Read the model definition and answer for the solid it produces. Units are mm, in the model's axes. A direction names the side the tool comes from. Coordinates: 2 decimals unless noted, no trailing zeros. Loops run counter-clockwise (first coordinate to the right, second up) from the corner with the lowest first, then second, coordinate; pieces in that order, holes last. Notation, with made-up numbers: (-25, -24) - (-2, -24) arc R4 ccw to (-2, -20) - close; hole circle Ø4 at (-2.75, -7). An arc over 180 degrees is marked (long way). One line per item, written item: value. Start each with the question number.
from build123d import *

# Parameters (mm, degrees)
SKETCH_1_W          = 41.5
SKETCH_1_H          = 16
EXTRUDE_1_DEPTH     = 28.5
FILLET_1_R          = 1
FILLET_2_R          = 0.5
CUT_EXTRUDE_START   = -0.5
CUT_EXTRUDE_1_DEPTH = 0.5
SKETCH_4_R          = 0.5
EXTRUDE_2_DEPTH     = 6


with BuildPart() as part:
    # Эскиз1 → Бобышка-Вытянуть1 (new body)
    with BuildSketch(Plane(origin=(0, 0, 0), x_dir=(1, 0, 0), z_dir=(0, 1, 0))):
        Rectangle(SKETCH_1_W, SKETCH_1_H)
    extrude(amount=EXTRUDE_1_DEPTH)

    # Скругление1
    fillet_1_edges = [part.edges().sort_by_distance(p)[0] for p in [
        (20.75, 14.25, 8),
        (-20.75, 14.25, 8),
        (-20.75, 14.25, -8),
        (20.75, 14.25, -8),
    ]]
    fillet(fillet_1_edges, radius=FILLET_1_R)

    # Скругление2
    fillet_2_edges = [part.edges().sort_by_distance(p)[0] for p in [
        (0, 28.5, -8),
        (20.75, 28.5, 0),
        (-20.75, 28.5, 0),
        (0, 28.5, 8),
        (-20.457106781, 28.5, 7.707106781),
        (-20.457106781, 28.5, -7.707106781),
        (20.457106781, 28.5, 7.707106781),
        (20.457106781, 28.5, -7.707106781),
    ]]
    fillet(fillet_2_edges, radius=FILLET_2_R)

    # Эскиз3 → Вырез-Вытянуть1 (cut)
    with BuildSketch(Plane.XZ.offset(CUT_EXTRUDE_START)):
        with BuildLine():
            Line((-10.920111581, 7.5), (-10.920111581, 8))
            Line((-10.920111581, 8), (-19.75, 8))
            ThreePointArc((-19.75, 8), (-20.457106781, 7.707106781), (-20.75, 7))
            Line((-20.75, 7), (-20.75, -7))
            ThreePointArc((-20.75, -7), (-20.457106781, -7.707106781), (-19.75, -8))
            Line((-19.75, -8), (-10.920111581, -8))
            Line((-10.920111581, -8), (-10.920111581, -7.5))
            Line((-10.920111581, -7.5), (-8.050796548, -7.5))
            Line((-8.050796548, -7.5), (-8.050796548, -8))
            Line((-8.050796548, -8), (8.050796548, -8))
            Line((8.050796548, -8), (8.050796548, -7.5))
            Line((8.050796548, -7.5), (10.920111581, -7.5))
            Line((10.920111581, -7.5), (10.920111581, -8))
            Line((10.920111581, -8), (19.75, -8))
            ThreePointArc((19.75, -8), (20.457106781, -7.707106781), (20.75, -7))
            Line((20.75, -7), (20.75, 7))
            ThreePointArc((20.75, 7), (20.457106781, 7.707106781), (19.75, 8))
            Line((19.75, 8), (10.920111581, 8))
            Line((10.920111581, 8), (10.920111581, 7.5))
            Line((10.920111581, 7.5), (8.050796548, 7.5))
            Line((8.050796548, 7.5), (8.050796548, 8))
            Line((8.050796548, 8), (-8.050796548, 8))
            Line((-8.050796548, 8), (-8.050796548, 7.5))
            Line((-8.050796548, 7.5), (-10.920111581, 7.5))
        make_face()
    extrude(amount=CUT_EXTRUDE_1_DEPTH, mode=Mode.SUBTRACT)

    # Эскиз4 → Бобышка-Вытянуть2 (add)
    with BuildSketch(Plane.XZ.offset(-0.5)):
        with Locations(Location((-18.75, 0, 0), (0, 0, 270))):
            Circle(SKETCH_4_R)
        with Locations(Location((18.75, 0, 0), (0, 0, 270))):
            Circle(SKETCH_4_R)
    extrude(amount=EXTRUDE_2_DEPTH)


solid = part.part
1) Section D-D, the plane x = 2.5 is taken. Determine the outline of the cut face in (y, z).
2) Section B-B, the plane x = 10 is taken. Determine the outline of the cut face in (y, z).
3) Flat-ended cylindrical pins translate along their axes: P1, Ø0.6, axis at x = 9.5, z = -7.5, coming from the -Y side; P2, Ø0.6, axis at y = 0.5, z = -8, coming from the -X side; P3, Ø3, axis at x = 2.5, z = 4, coming from the -Y side. Find the tip coordinate at first contact, or state that the pin passes through.
4) Section A-A, the plane z = 0 is taken. Determine the outline of the cut face in (x, y), and give its area (3 significant figures).
5) For faces 4 (the flat face through (19, -5.5, 0)), 5 (the cylindrical face through (-18.254, -2.458, 0.065)), determine the directions among +Z, -Z, +X, -X, +Y, -Y from which every point of the face is accessible in a straight line to the end or side of a thin tool.
6) Determine the mould class of faces 1 (the flat face through (-20.75, 14, 0)), 2 (the flat face through (0, 0.5, 0)), 3 (the cylindrical face through (20.465, 14.442, -7.699)) for opening direction Z: released by +Z, released by -Z, zero draft, split by the parting line, or undercut.
7) Section C-C, the plane y = -3 is taken. Determine the outline of the cut face in (x, z).
8) Straight lines are drawn through the part: L1, parallel to Y at x = -12, z = 2; L2, parallel to X at y = 6.5, z = 7.25. For each, find the intervals that lie inside material, in ascending order.
Answer below:
1. outline: (0.5, -8) - (28, -8) arc R0.5 ccw to (28.5, -7.5) - (28.5, 7.5) arc R0.5 ccw to (28, 8) - (0.5, 8) - close
2. outline: (0, -8) - (28, -8) arc R0.5 ccw to (28.5, -7.5) - (28.5, 7.5) arc R0.5 ccw to (28, 8) - (0, 8) - (0, 7.5) - (0.5, 7.5) - (0.5, -7.5) - (0, -7.5) - close
3. P1: y = 0
3. P2: x = -20.46
3. P3: y = 0.5
4. outline: (-20.75, 0.5) - (-19.25, 0.5) - (-19.25, -5.5) - (-18.25, -5.5) - (-18.25, 0.5) - (18.25, 0.5) - (18.25, -5.5) - (19.25, -5.5) - (19.25, 0.5) - (20.75, 0.5) - (20.75, 28) arc R0.5 ccw to (20.25, 28.5) - (-20.25, 28.5) arc R0.5 ccw to (-20.75, 28) - close
4. area: 1,170 mm2
5. face 4: +Z, -Z, +X, -X, -Y
5. face 5: -Y
6. face 1: zero draft
6. face 2: undercut
6. face 3: released by -Z
7. outline: circle Ø1 at (-18.75, 0); circle Ø1 at (18.75, 0)
8. L1: 0.5 to 28.5
8. L2: -20.72 to 20.72
